Verification items for the finished model (mm, model axes). A direction names the side the tool comes from. Give positions to 0.01 mm unless a question says otherwise; leave off trailing zeros. Order: outer loops, then holes, each group sorted by start corner. A loop starts at its lowest first (then second) coordinate and runs counter-clockwise, first axis right, second up. Notation, with made-up numbers: (72.25, -25.75) -> (131.25, -25.75) arc R13 ccw to (131.25, -1.75) -> close; hole circle Ø8 at (-14.5, 66). An arc over 180 degrees is marked (long way). Return JSON: item names as keys, results as strings. Group by question number.
(1) Depth check by flat-ended pin: pin 1 Ø1 at (y, z) = (-3.5, 23.5) entering from -X; pin 2 Ø1 at (y, z) = (2, 49.5) entering from +X; pin 3 Ø1.5 at (x, z) = (6.5, 51.5) entering from +Y. Enter the tip coordinate at first touch or a pass-through.
(2) Cross-section at D-D on x = 5. Enter the section's corners in (y, z).
(3) Cross-section at B-B on z = 50. Enter the section's corners in (x, y).
(4) Tool access check on faces 1 (the face through (0, 10, 43)), 2 (the face through (0, 0, 66.2)). Record the directions out of +Z, -Z, +X, -X, +Y, -Y that give a thin tool (end or side, any length) a straight path to the whole face; none if there is none.
(5) Thickness scan on line 1 along Z through (x, y) = (5, 8.5); line 2 along X through (y, z) = (-6, 50); line 3 along X through (y, z) = (9.25, 4). Record the ranges inside material, lowest first.
(6) Cross-section at C-C on y = -1.75. Enter the section's corners in (x, z).
(7) Cross-section at A-A on x = 0. Enter the section's corners in (y, z), then the cut area to 3 significant figures.
from build123d import *

# Parameters (mm, degrees)
EXTRUDE_3_DEPTH = 43
SKETCH_3_R      = 9.2
EXTRUDE_4_DEPTH = 66.2


with BuildPart() as part:
    # 草图1 → 凸台-拉伸3 (new body)
    with BuildSketch(Plane.XY):
        with BuildLine():
            Line((-3, 12.2), (3, 12.2))
            Line((3, 12.2), (7.692674554, 5.046063634))
            ThreePointArc((7.692674554, 5.046063634), (0, -9.2), (-7.692674554, 5.046063634))
            Line((-7.692674554, 5.046063634), (-3, 12.2))
        make_face()
    extrude(amount=EXTRUDE_3_DEPTH)

    # 草图3 → 凸台-拉伸4 (add)
    with BuildSketch(Plane(origin=(0, 0, 0), x_dir=(-1, 0, 0), z_dir=(0, 0, -1))):
        Circle(SKETCH_3_R)
    extrude(amount=-EXTRUDE_4_DEPTH)


solid = part.part
Verdict:
{
 "1": {"pin 1": "x = -8.7", "pin 2": "x = 9.08", "pin 3": "y = 7.18"},
 "2": {"outline": "(-7.72, 0) -> (9.15, 0) -> (9.15, 43) -> (7.72, 43) -> (7.72, 66.2) -> (-7.72, 66.2) -> close"},
 "3": {"outline": "circle Ø18.4 at (0, 0)"},
 "4": {"face 1": "+Z, +Y", "face 2": "+Z, +X, -X, +Y, -Y"},
 "5": {"line 1": "0 to 43", "line 2": "-6.97 to 6.97", "line 3": "-4.94 to 4.94"},
 "6": {"outline": "(-9.03, 0) -> (9.03, 0) -> (9.03, 66.2) -> (-9.03, 66.2) -> close"},
 "7": {"outline": "(-9.2, 0) -> (12.2, 0) -> (12.2, 43) -> (9.2, 43) -> (9.2, 66.2) -> (-9.2, 66.2) -> close", "area": "1,350 mm²"}
}
